```python
from build123d import *

# Parameters (mm, degrees)
BOSS_EXTRUDE1_OUTLINE_R = 1.75
BOSS_EXTRUDE1_DEPTH     = 4
CUT_EXTRUDE1_DEPTH      = 1


# Read off the part's stored shape, not the designer's step: Boss-Extrude1
with BuildPart() as part:
    # Boss-Extrude1 outline → Boss-Extrude1 (new body)
    with BuildSketch(Plane(origin=(0, 0, 0), x_dir=(1, 0, 0), z_dir=(0, 1, 0))):
        with BuildLine():
            Line((47.379776182, -18.81631662), (60.379776182, -18.81631662))
            Line((60.379776182, -18.81631662), (60.379776182, -4.977921711))
            Line((60.379776182, -4.977921711), (-19.620223818, -4.977921711))
            Line((-19.620223818, -4.977921711), (-19.620223818, -18.81631662))
            Line((-19.620223818, -18.81631662), (-6.620223818, -18.81631662))
            Line((-6.620223818, -18.81631662), (-6.620223818, -10.33744254))
            Line((-6.620223818, -10.33744254), (7.44307775, -10.33744254))
            ThreePointArc((7.44307775, -10.33744254), (9.879776182, -5.587442326), (12.316474615, -10.33744254))
            Line((12.316474615, -10.33744254), (21.44307775, -10.33744254))
            ThreePointArc((21.44307775, -10.33744254), (23.879776183, -5.587442326), (26.316474615, -10.33744254))
            Line((26.316474615, -10.33744254), (35.44307775, -10.33744254))
            ThreePointArc((35.44307775, -10.33744254), (37.879776183, -5.587442326), (40.316474615, -10.33744254))
            Line((40.316474615, -10.33744254), (47.379776182, -10.33744254))
            Line((47.379776182, -10.33744254), (47.379776182, -18.81631662))
        make_face()
        with Locations((-14.620223818, -13.58744255)):
            Circle(BOSS_EXTRUDE1_OUTLINE_R, mode=Mode.SUBTRACT)
        with Locations((55.379776182, -13.58744255)):
            Circle(BOSS_EXTRUDE1_OUTLINE_R, mode=Mode.SUBTRACT)
    extrude(amount=BOSS_EXTRUDE1_DEPTH)

    # Sketch2 → Cut-Extrude1 (cut)
    with BuildSketch(Plane(origin=(0, 4, 0), x_dir=(1, 0, 0), z_dir=(0, 1, 0))):
        Polygon((-15.320752279, -6.539659084), (-13.773957408, -6.539659084), (-13.773957408, -7.109530878), (-14.750880484, -7.109530878), (-14.750880484, -7.720107802), (-13.773957408, -7.720107802), (-13.773957408, -8.289979596), (-14.750880484, -8.289979596), (-14.750880484, -9.714659084), (-15.320752279, -9.714659084), align=None)
        Polygon((-12.863816182, -6.539659084), (-11.982931767, -6.539659084), (-11.982931767, -9.714659084), (-12.552803561, -9.714659084), (-12.552803561, -7.06882575), (-13.204085613, -7.06882575), align=None)
    extrude(amount=-CUT_EXTRUDE1_DEPTH, mode=Mode.SUBTRACT)


solid = part.part
```
Input: part model. Units: mm. Frame: model coordinates. A direction names the side the tool comes from. Give positions to 0.01 mm unless a question says otherwise; leave off trailing zeros. Loops run counter-clockwise (first coordinate to the right, second up) from the corner with the lowest first, then second, coordinate; pieces in that order, holes last. Notation, with made-up numbers: (75.25, 85.25) -> (96.25, 85.25) arc R26 cw to (96.25, 110.25) -> close; hole circle Ø4 at (9, 19.25). An arc over 180 degrees is marked (long way). Use a Markdown table: item, result.
Q1. Access query for faces 1 (the flat face through (44, 2, 10.337)), 2 (the flat face through (20, 0, 10)). Directions: +Z, -Z, +X, -X, +Y, -Y. A direction counts if a zero-diameter tool reaches every point of the face in a straight line with its end or side. Return the directions, or none.
Entries:
| item | result |
|---|---|
| face 1 | +Z, +Y, -Y |
| face 2 | +Z, -Z, +X, -X, -Y |
Q2. Section query C-C, the plane z = 12.75. Return the cut outline in (x, y), plus the area to 3 significant figures.
Entries:
| item | result |
|---|---|
| outline | (-19.62, 0) -> (-16.16, 0) -> (-16.16, 4) -> (-19.62, 4) -> close; (-13.08, 0) -> (-6.62, 0) -> (-6.62, 4) -> (-13.08, 4) -> close; (47.38, 0) -> (53.84, 0) -> (53.84, 4) -> (47.38, 4) -> close; (56.92, 0) -> (60.38, 0) -> (60.38, 4) -> (56.92, 4) -> close |
| area | 79.4 mm² |
Q3. Section query D-D, the plane x = 43. Return the cut outline in (y, z).
Entries:
| item | result |
|---|---|
| outline | (0, 4.98) -> (4, 4.98) -> (4, 10.34) -> (0, 10.34) -> close |
Q4. Pull-direction query (Z, two-part tool) for faces 3 (the flat face through (31, 2, 10.337)), 4 (the flat face through (20, 4, 10)), 5 (the cylindrical face through (-15, 1.972, 15.296)); classes: pulls with the +Z half, pulls with the -Z half, needs draft (parallel to the pull), parting line crosses it, or undercut.
Entries:
| item | result |
|---|---|
| face 3 | pulls with the +Z half |
| face 4 | needs draft |
| face 5 | undercut |
Q5. Section query B-B, the plane y = 2.2. Return the cut outline in (x, z).
Entries:
| item | result |
|---|---|
| outline | (-19.62, 4.98) -> (60.38, 4.98) -> (60.38, 18.82) -> (47.38, 18.82) -> (47.38, 10.34) -> (40.32, 10.34) arc R3 cw (long way) to (35.44, 10.34) -> (26.32, 10.34) arc R3 cw (long way) to (21.44, 10.34) -> (12.32, 10.34) arc R3 cw (long way) to (7.44, 10.34) -> (-6.62, 10.34) -> (-6.62, 18.82) -> (-19.62, 18.82) -> close; hole circle Ø3.5 at (-14.62, 13.59); hole circle Ø3.5 at (55.38, 13.59) |
Q6. Section query A-A, the plane z = 17.25. Return the cut outline in (x, y), plus the area to 3 significant figures.
Entries:
| item | result |
|---|---|
| outline | (-19.62, 0) -> (-6.62, 0) -> (-6.62, 4) -> (-19.62, 4) -> close; (47.38, 0) -> (60.38, 0) -> (60.38, 4) -> (47.38, 4) -> close |
| area | 104 mm² |
Q7. Ray query, probe 1 along X at (y, z) = (1.95, 13.5); probe 2 along X at (y, z) = (2.35, 8.75); probe 3 along X at (y, z) = (0.7, 15.5). Return the intervals inside material, ascending. Write a range as from..to.
Entries:
| item | result |
|---|---|
| probe 1 | x = -19.62..-16.37, -12.87..-6.62, 47.38..53.63, 57.13..60.38 |
| probe 2 | x = -19.62..6.88, 12.88..20.88, 26.88..34.88, 40.88..60.38 |
| probe 3 | x = -19.62..-6.62, 47.38..60.38 |
